Geometry: see drawing. Coordinates: mm, zero at the bounding-box minimum. A direction names the side the tool comes from. Round coordinates to 2 decimals unless told otherwise and drop trailing zeros. Loops run counter-clockwise (first coordinate to the right, second up) from the corner with the lowest first, then second, coordinate; pieces in that order, holes last. Notation, with made-up numbers: (39, 5.5) - (71, 5.5) arc R32 ccw to (71, 41.5) - close; hole circle Ø11 at (-19.75, 44.25). An arc over 180 degrees is marked (long way). Return JSON: item names as keys, results as strings. Group by question number.
1. Draft query along X for the marked faces 3, 4 and 5. Return one class per face: +X half, -X half, draft (parallel to the pull), parting line (faces both ways), or undercut.
2. Section C-C on z = 12. Return loops of the section in (x, y).
3. Section D-D on x = 6.75. Return loops of the section in (y, z), and give its area (3 significant figures).
4. Set-up query: the marked faces 1 and 2. Return all of +Z, -Z, +X, -X, +Y, -Y with unobstructed straight access to the full face (end or side cutting, diameter ignored); none if empty.
5. Material intervals for probe 1 along Y at (x, z) = (11, 16); probe 2 along X at (y, z) = (7.7, 2.5) (3 decimals); probe 3 along Y at (x, z) = (11.2, 7) (3 decimals), sorted ascending.
6. First-contact query: pin 1 Ø8 at (y, z) = (8, 15) entering from -X; pin 2 Ø2 at (x, y) = (4.5, 6) entering from +Z; pin 3 Ø3.5 at (x, y) = (8.5, 7.5) entering from +Z. Flat tips, straight axial feed; report the tip coordinate or a pass-through.
7. Section B-B on x = 11.2. Return loops of the section in (y, z) (3 decimals), and give its area (3 significant figures).
8. Section A-A on y = 7.7. Return loops of the section in (x, z) (3 decimals).
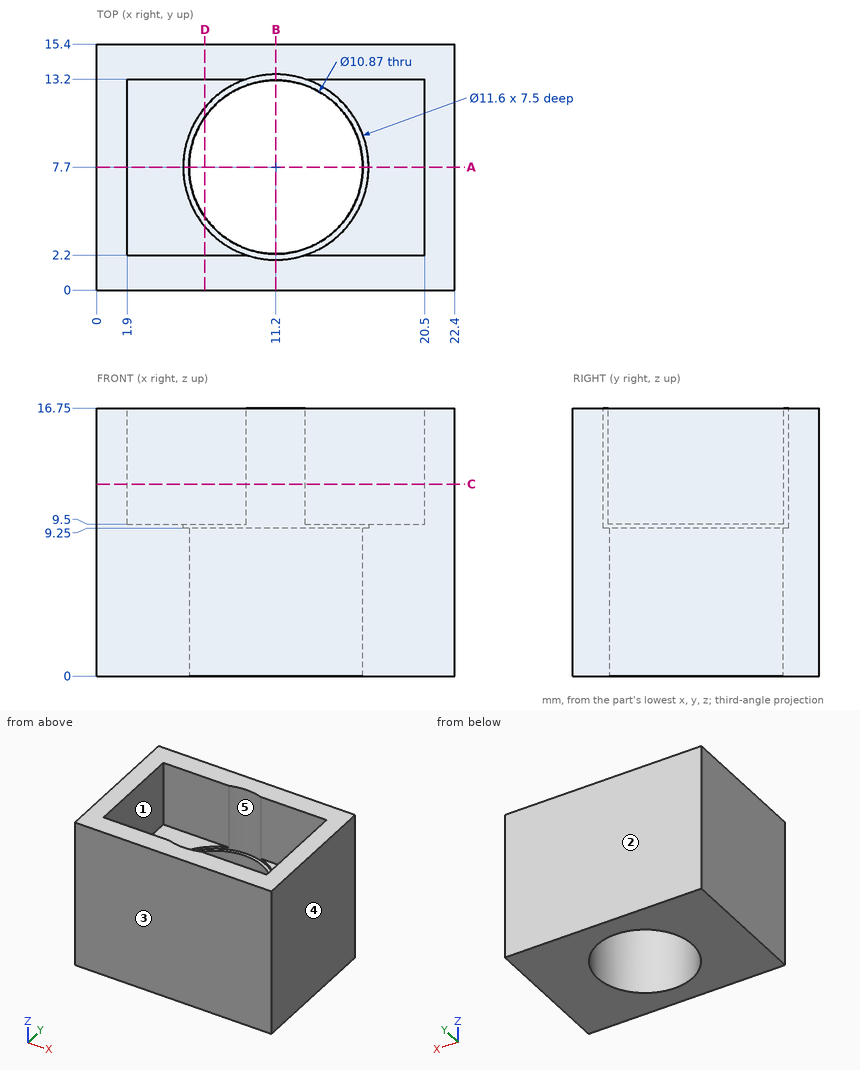
Taken from the geometry:
{
 "1": {"face 3": "draft", "face 4": "+X half", "face 5": "undercut"},
 "2": {"outline": "(0, 0) - (22.4, 0) - (22.4, 15.4) - (0, 15.4) - close; hole (1.9, 2.2) - (9.36, 2.2) arc R5.8 ccw to (13.04, 2.2) - (20.5, 2.2) - (20.5, 13.2) - (13.04, 13.2) arc R5.8 ccw to (9.36, 13.2) - (1.9, 13.2) - close"},
 "3": {"outline": "(0, 0) - (4.58, 0) - (4.58, 9.25) - (3.98, 9.25) - (3.98, 9.5) - (2.2, 9.5) - (2.2, 16.75) - (0, 16.75) - close; (10.82, 0) - (15.4, 0) - (15.4, 16.75) - (13.2, 16.75) - (13.2, 9.5) - (11.42, 9.5) - (11.42, 9.25) - (10.82, 9.25) - close", "area": "119 mm2"},
 "4": {"face 1": "+Z", "face 2": "+Z, -Z, +X, -X, +Y"},
 "5": {"probe 1": "0 to 1.9, 13.5 to 15.4", "probe 2": "0 to 5.765, 16.635 to 22.4", "probe 3": "0 to 2.265, 13.135 to 15.4"},
 "6": {"pin 1": "x = 0", "pin 2": "z = 9.5", "pin 3": "through"},
 "7": {"outline": "(0, 0) - (2.265, 0) - (2.265, 9.25) - (1.9, 9.25) - (1.9, 16.75) - (0, 16.75) - close; (13.135, 0) - (15.4, 0) - (15.4, 16.75) - (13.5, 16.75) - (13.5, 9.25) - (13.135, 9.25) - close", "area": "70.4 mm2"},
 "8": {"outline": "(0, 0) - (5.765, 0) - (5.765, 9.25) - (5.4, 9.25) - (5.4, 9.5) - (1.9, 9.5) - (1.9, 16.75) - (0, 16.75) - close; (16.635, 0) - (22.4, 0) - (22.4, 16.75) - (20.5, 16.75) - (20.5, 9.5) - (17, 9.5) - (17, 9.25) - (16.635, 9.25) - close"}
}
